Autodesk Inventor part; units mm, degrees
ref_plane "YZ Plane" through (0, 0, 0) normal (1, 0, 0) x (0, 1, 0)
ref_plane "XZ Plane" through (0, 0, 0) normal (0, 1, 0) x (-1, 0, 0)
ref_plane "XY Plane" through (0, 0, 0) normal (0, 0, 1) x (1, 0, 0)
sketch "Sketch1" plane through (0, 0, 0) normal (0, 1, 0) x (-1, 0, 0)
  line L0 (12, 7.85) -> (-12, 7.85)
  line L1 (-14, 5.85) -> (-14, -5.85)
  line L2 (-12, -7.85) -> (12, -7.85)
  line L3 (14, -5.85) -> (14, 5.85)
  line L4 (14, 7.85) -> (-14, -7.85) construction
  line L5 (-14, 7.85) -> (14, -7.85) construction
  arc A0 (14, 5.85) -> (12, 7.85) centre (12, 5.85) ccw
  arc A1 (12, -7.85) -> (14, -5.85) centre (12, -5.85) ccw
  arc A2 (-14, -5.85) -> (-12, -7.85) centre (-12, -5.85) ccw
  arc A3 (-12, 7.85) -> (-14, 5.85) centre (-12, 5.85) ccw
  line L6 (12.5, 8.7909) -> (12.5, -11.3064) construction
  line L7 (15.2914, 6.35) -> (1.3637, 6.35) construction
  circle A4 centre (11, 4.85) radius 1.5
  line L8 (14, 0) -> (-14, 0) construction
  line L9 (0, 7.85) -> (0, -7.85) construction
  circle A5 centre (-11.135, -4.985) radius 1.5
  point P0 (0, 0)
  dimension "d0" = 28
  dimension "d1" = 15.7
  dimension "d2" = 2
  dimension "d3" = 1.5
  dimension "d4" = 1.5
  dimension "d5" = 3
  dimension "d15" = 3
extrude "Extrusion1" add sketch "Sketch1" along normal blind 9.7
sketch "Sketch2" plane through (-12, 0, 7.85) normal (0, 0, 1) x (1, 0, 0)
  line L0 (0, 0) -> (24, 0) construction
  line L1 (24, 0) -> (24, 9.7) construction
  line L2 (0, 9.7) -> (24, 9.7) construction
  line L3 (0, 0) -> (0, 9.7) construction
  line L4 (0, 6.7) -> (24, 6.7) construction
  line L5 (24, 0) -> (24, 9.7) construction
  line L6 (0, 9.7) -> (24, 9.7) construction
  line L7 (23.5, 9.7) -> (23.5, 0) construction
  line L8 (0, 0) -> (24, 0) construction
  line L9 (26, 0) -> (26, 9.7) construction
  line L10 (23.5, 6.7) -> (20.7, 6.7)
  line L11 (20.7, 6.7) -> (20.7, 2.8)
  line L12 (20.7, 2.8) -> (23.5, 2.8)
  line L13 (23.5, 2.8) -> (23.5, 6.7)
  point P0 (12, 0)
  dimension "d8" = 3
  dimension "d9" = 2.5
  dimension "d10" = 2.8
  dimension "d11" = 3.9
extrude "Extrusion2" add sketch "Sketch2" along normal blind 2.3
fillet "Fillet1" radius 1 2 edges at (8.7, 4.75, 10.15) (11.5, 4.75, 10.15)
properties part number "microswitch" material "PET Plastic"
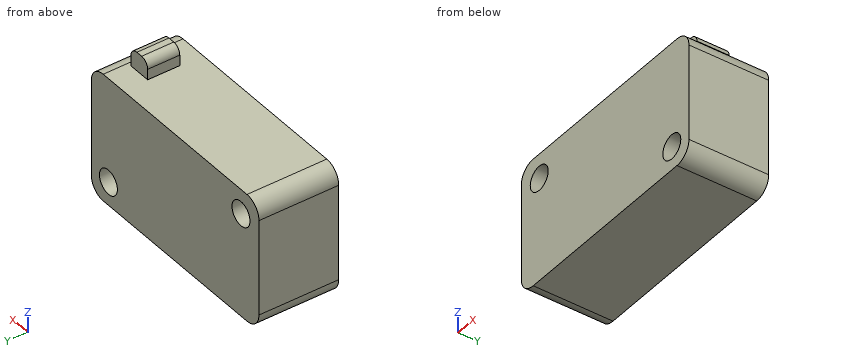
Model file for the job. Use its own axes, mm. Give positions to 0.01 mm unless a question says otherwise; leave off trailing zeros. Order: outer loops, then holes, each group sorted by start corner. A loop starts at its lowest first (then second) coordinate and runs counter-clockwise, first axis right, second up. Notation, with made-up numbers: (13.5, 24) - (22.5, 24) arc R13 ccw to (22.5, 34) - close; hole circle Ø5 at (-18, 29). An arc over 180 degrees is marked (long way). Return JSON: item names as keys, results as strings.
1) Cut at C-C, the plane y = 7. Give the cut face in (x, z) (3 decimals), plus the area to 3 significant figures.
Geometry says:
{"outline": "(-14, -5.85) arc R2 ccw to (-12, -7.85) - (12, -7.85) arc R2 ccw to (14, -5.85) - (14, 5.85) arc R2 ccw to (12, 7.85) - (-12, 7.85) arc R2 ccw to (-14, 5.85) - close; hole circle Ø3 at (-11, 4.85); hole circle Ø3 at (11.135, -4.985)", "area": "422 mm²"}
2) Cut at A-A, the plane x = -11. Give the cut face in (y, z), plus the area to 3 significant figures.
Geometry says:
{"outline": "(0, -7.85) - (9.7, -7.85) - (9.7, 3.35) - (0, 3.35) - close; (0, 6.35) - (9.7, 6.35) - (9.7, 7.85) - (0, 7.85) - close", "area": "123 mm²"}
3) Probe line 1 (Z direction, x = -11, y = 2.5); line 2 (Z direction, x = -7, y = 3.25); line 3 (Z direction, x = 11, y = 5.25). List the from-to ranges inside material, lowest first. Write a range as from..to.
Geometry says:
{"line 1": "-7.85..3.35, 6.35..7.85", "line 2": "-7.85..7.85", "line 3": "-7.85..-6.48, -3.49..10.02"}
4) Cut at D-D, the plane x = -3.25. Give the cut face in (y, z), plus the area to 3 significant figures.
Geometry says:
{"outline": "(0, -7.85) - (9.7, -7.85) - (9.7, 7.85) - (0, 7.85) - close", "area": "152 mm²"}
5) Cut at B-B, the plane z = 4.85. Give the cut face in (x, y), plus the area to 4 significant figures.
Geometry says:
{"outline": "(-14, 0) - (-12.5, 0) - (-12.5, 9.7) - (-14, 9.7) - close; (-9.5, 0) - (14, 0) - (14, 9.7) - (-9.5, 9.7) - close", "area": "242.5 mm²"}
6) Flat gauge pins, fed straight in: P1, Ø0.7, axis at y = 4, z = 8, coming from the -X side; P2, Ø0.7, axis at y = 5.5, z = 8.5, coming from the +X side; P3, Ø1.8, axis at x = -11, z = 4.85, coming from the +Y side; P4, Ø0.7, axis at x = 9.5, z = 8.5, coming from the +Y side. Where does each tip first touch, or does it go through?
Geometry says:
{"P1": "x = -12.87", "P2": "x = 11.5", "P3": "through", "P4": "y = 6.7"}
